Could you check a few things on this model? Use its own coordinates, in mm. Give positions to 0.01 mm unless a question says otherwise; leave off trailing zeros. Loops run counter-clockwise (first coordinate to the right, second up) from the corner with the lowest first, then second, coordinate; pieces in that order, holes last. Notation, with made-up numbers: (26, 71.5) -> (57, 71.5) arc R13 ccw to (57, 93.5) -> close; hole circle Ø7 at (-27.5, -15). An arc over 180 degrees is marked (long way). Write each question's results on one line, items separated by ' | '. Start each with the question number.
Q1. If we section it at D-D, the plane y = 2: List the corners of the cut face in (x, z) for me.
Q2. If I drill on line 1 along X through (y, z) = (0.6, 0); line 2 along Z through (x, y) = (0, 2.2); line 3 along Y through (x, z) = (11, 1), over which ranges is the centre line in solid material (lowest first)?
Q3. If we section it at A-A, the plane y = 1.1: List the corners of the cut face in (x, z) for me.
Q4. Will these pins go through, and if not, where does the flat tip stop? P1, Ø3, axis at x = 12.5, z = 0, coming from the +Y side; P2, Ø1, axis at x = -0.5, y = 2.5, coming from the +Z side; P3, Ø1.5, axis at x = 3, y = 1, coming from the +Z side.
Q5. If we section it at C-C, the plane x = 12.5: List the corners of the cut face in (y, z) for me, plus the area to 3 significant figures.
Q6. We'd pull the mould along X, two halves only. Please class faces 1 (the face through (2, 3.8, 2)), 2 (the face through (2.204, 1.451, 1.179)), 3 (the face through (9.272, 0.74, -1.834)): released by +X, released by -X, zero draft, split by the parting line, or undercut.
from build123d import *

# Parameters (mm, degrees)
SKETCH1_R                 = 2.5
SKETCH1_R_2               = 1
BOSS_EXTRUDE1_DEPTH       = 1.5
BOSS_EXTRUDE2_START       = 1.5
BOSS_EXTRUDE2_OUTLINE_R   = 3.5
BOSS_EXTRUDE2_OUTLINE_R_2 = 2.5
BOSS_EXTRUDE2_DEPTH       = 2.3


# Read off the part's stored shape, not the designer's step: Boss-Extrude2
with BuildPart() as part:
    # Sketch1 → Boss-Extrude1 (new body)
    with BuildSketch(Plane(origin=(0, 0, 0), x_dir=(1, 0, 0), z_dir=(0, 1, 0))):
        with BuildLine():
            ThreePointArc((2.227105745, 2.7), (-3.5, 0), (2.227105745, -2.7))
            Line((2.227105745, -2.7), (16.121967257, -0.992534124))
            ThreePointArc((16.121967257, -0.992534124), (17, 0), (16.121967257, 0.992534124))
            Line((16.121967257, 0.992534124), (2.227105745, 2.7))
        make_face()
        with Locations(Location((0, 0, 0), (0, 0, 270))):
            Circle(SKETCH1_R, mode=Mode.SUBTRACT)
        with Locations(Location((12.5, 0, 0), (0, 0, 270))):
            Circle(SKETCH1_R_2, mode=Mode.SUBTRACT)
    extrude(amount=BOSS_EXTRUDE1_DEPTH)

    # Boss-Extrude2 outline → Boss-Extrude2 (add)
    with BuildSketch(Plane(origin=(0, 0, 0), x_dir=(1, 0, 0), z_dir=(0, 1, 0)).offset(BOSS_EXTRUDE2_START)):
        Circle(BOSS_EXTRUDE2_OUTLINE_R)
        Circle(BOSS_EXTRUDE2_OUTLINE_R_2, mode=Mode.SUBTRACT)
    extrude(amount=BOSS_EXTRUDE2_DEPTH)


solid = part.part
Final values:
1) outline: circle Ø7 at (0, 0); hole circle Ø5 at (0, 0)
2) line 1: x = -3.5 to -2.5, 2.5 to 11.5, 13.5 to 17 | line 2: z = -3.5 to -2.5, 2.5 to 3.5 | line 3: y = 0 to 1.5
3) outline: (2.23, -2.7) -> (16.12, -0.99) arc R1 ccw to (16.12, 0.99) -> (2.23, 2.7) arc R3.5 ccw (long way) to start; hole circle Ø5 at (0, 0); hole circle Ø2 at (12.5, 0)
4) P1: stops at y = 1.5 | P2: stops at z = 3.5 | P3: stops at z = 2.7
5) outline: (0, -1.44) -> (1.5, -1.44) -> (1.5, -1) -> (0, -1) -> close; (0, 1) -> (1.5, 1) -> (1.5, 1.44) -> (0, 1.44) -> close | area: 1.31 mm²
6) face 1: zero draft | face 2: undercut | face 3: released by +X
